```python
from build123d import *

# Parameters (mm, degrees)
SKETCH1_R           = 6.171386398
BOSS_EXTRUDE1_DEPTH = 9.525
CUT_EXTRUDE1_DEPTH  = 9.525
CUT_EXTRUDE2_DEPTH  = 9.525
CUT_EXTRUDE3_DEPTH  = 9.525
SKETCH3_R           = 6.35
CUT_EXTRUDE4_DEPTH  = 9.525


with BuildPart() as part:
    # Sketch1 → Boss-Extrude1 (new body)
    with BuildSketch(Plane.XY):
        Polygon((0, 0), (53.773244147, 21.40735786), (103.498996656, 0), (119.524414716, -130.99264214), (69.064214047, -130.99264214), align=None)
        with Locations((53.773244147, 0)):
            Circle(SKETCH1_R, mode=Mode.SUBTRACT)
    extrude(amount=BOSS_EXTRUDE1_DEPTH)

    # Sketch2 → Cut-Extrude1 (cut)
    with BuildSketch(Plane.XY.offset(9.525)):
        Polygon((46.017470702, 18.319751369), (37.167957105, 14.79672226), (38.342300142, 11.846884394), (47.191813738, 15.369913504), align=None)
        Polygon((31.858248947, 12.682904794), (23.008735351, 9.159875685), (24.183078387, 6.210037819), (33.032591984, 9.733066929), align=None)
        Polygon((17.699027193, 7.046058219), (8.849513596, 3.523029109), (10.023856633, 0.573191244), (18.873370229, 4.096220353), align=None)
    extrude(amount=-CUT_EXTRUDE1_DEPTH, mode=Mode.SUBTRACT)

    # Sketch2_3 → Cut-Extrude2 (cut)
    with BuildSketch(Plane.XY.offset(9.525)):
        Polygon((7.250861941, -6.944872289), (4.44231406, -8.425643642), (8.884628121, -16.851287285), (11.693176002, -15.370515931), align=None)
        Polygon((20.637034977, -32.334145131), (17.828487096, -33.814916485), (22.270801156, -42.240560127), (25.079349037, -40.759788774), align=None)
        Polygon((34.023208012, -57.723417974), (31.214660132, -59.204189327), (35.656974192, -67.629832969), (38.465522073, -66.149061616), align=None)
        Polygon((47.409381048, -83.112690816), (44.600833167, -84.593462169), (49.043147228, -93.019105812), (51.851695108, -91.538334458), align=None)
        Polygon((60.795554083, -108.501963658), (57.987006203, -109.982735012), (62.429320263, -118.408378654), (65.237868144, -116.927607301), align=None)
    extrude(amount=-CUT_EXTRUDE2_DEPTH, mode=Mode.SUBTRACT)

    # Sketch2_4 → Cut-Extrude3 (cut)
    with BuildSketch(Plane.XY.offset(9.525)):
        Polygon((71.270661843, 13.874571258), (62.521952995, 17.640964559), (61.266488562, 14.724728276), (70.015197409, 10.958334976), align=None)
        Polygon((94.600552104, 3.83085579), (85.851843256, 7.597249091), (84.596378823, 4.681012808), (93.34508767, 0.914619507), align=None)
        Polygon((105.812294522, -18.909023057), (104.655645589, -9.454511529), (101.504141746, -9.840061173), (102.660790679, -19.294572702), align=None)
        Polygon((109.667790966, -50.424061486), (108.511142033, -40.969549957), (105.35963819, -41.355099602), (106.516287124, -50.80961113), align=None)
        Polygon((110.371783568, -82.324649559), (113.523287411, -81.939099915), (112.366638477, -72.484588386), (109.215134635, -72.870138031), align=None)
        Polygon((114.227280012, -113.839687988), (117.378783855, -113.454138344), (116.222134922, -103.999626815), (113.070631079, -104.385176459), align=None)
    extrude(amount=-CUT_EXTRUDE3_DEPTH, mode=Mode.SUBTRACT)

    # Sketch3 → Cut-Extrude4 (cut)
    with BuildSketch(Plane.XY.offset(9.525)):
        with Locations((94.294314381, -118.29264214)):
            Circle(SKETCH3_R)
    extrude(amount=-CUT_EXTRUDE4_DEPTH, mode=Mode.SUBTRACT)


solid = part.part
```
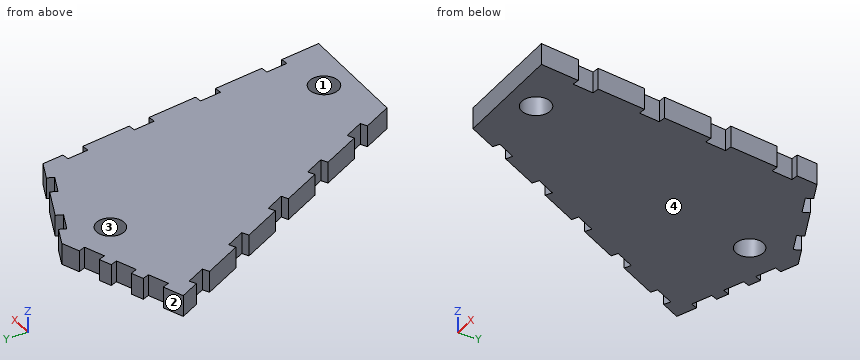
Read the model definition and answer for the solid it produces. Units are mm, in the model's axes. Face numbers are marked on the shaded views. Give positions to 0.01 mm unless a question says otherwise; leave off trailing zeros. Write each loop counter-clockwise with the first axis right and the second up, starting at its lowest first coordinate (ties: lowest second). Pieces come first, ordered by that corner, then holes. Notation, with made-up numbers: M 47.5,26 L 88.5,26 A13 ccw 88.5,34 Z; hole C 8,9.5 d10. An arc over 180 degrees is marked long. Put each result on its own line as item: value. Start each with the question number.
1. For a pull along Y with two mould halves and no side action, classify the marked faces 1, 2, 3 and 4 as released by +Y, released by -Y, zero draft, split by the parting line, or undercut.
2. Each of these flat-tipped pins is pushed along its axis until it touches: pin 1 Ø2 at (y, z) = (-111.5, 7.5) entering from -X; pin 2 Ø2 at (y, z) = (-34.5, 6) entering from +X. Where does it stop, or does it pass through?
3. Consider line 1 along Y through (x, z) = (51, 6.5); line 2 along X through (y, z) = (11.5, 7.5); line 3 along Y through (x, z) = (74, 7.25). Determine where each line is inside the solid, lowest interval first.
4. The part is cut by section B-B, the plane z = 5. Give the number of separate pieces and of enclosed holes in the cut face, and give its area (3 significant figures).
5. The part is cut by section A-A, the plane x = 14. Give the vertices of the cut face in (y, z) (1 decimal).
6. The part is cut by section C-C, the plane x = 76.5. Give the vertices of the cut face in (y, z) (3 decimals), and give its area (3 significant figures).
Final values:
1. face 1: undercut
1. face 2: released by +Y
1. face 3: undercut
1. face 4: zero draft
2. pin 1: stops at x = 61.85
2. pin 2: stops at x = 107.84
3. line 1: y = -96.73 to -91.99, -89.92 to -5.51, 5.51 to 20.3
3. line 2: x = 32.33 to 68.76, 70.25 to 76.79
3. line 3: y = -130.99 to 12.7
4. separate pieces: 1
4. enclosed holes: 2
4. area: 10,500 mm²
5. outline: M -26.6,0 L 2.2,0 L 2.2,9.5 L -26.6,9.5 Z
6. outline: M -130.993,0 L 11.623,0 L 11.623,9.525 L -130.993,9.525 Z
6. area: 1,360 mm²
